```python
from build123d import *

# Parameters (mm, degrees)
F0_W     = 88.9
F0_H     = 327.66
F0_R     = 12.7
F0_R_2   = 12.7063161154
F1_DEPTH = 0.5
F2_DEPTH = 0.005
F3_R     = 5.08
F4_R     = 5.08


# Not quite as in the source:
# - a feature names something its author has since deleted; it is built from what else it names


with BuildPart() as f1:
    # F0 (on Top) → F1 (new body)
    with BuildSketch(Plane.XY):
        with Locations((-16.0019993782, 26.0465461761)):
            Rectangle(F0_W, F0_H)
        with Locations((5.5880006218, -113.6534538239)):
            Circle(F0_R, mode=Mode.SUBTRACT)
        with Locations((-37.5932163954, 166.1064843748)):
            Circle(F0_R_2, mode=Mode.SUBTRACT)
        with BuildLine():
            ThreePointArc((5.589217639, 178.8128004902), (14.573939928, 175.0912066639), (18.2955337543, 166.1064843748))
            Line((18.2955337543, 166.1064843748), (18.2955337543, -96.8894538239))
            Line((18.2955337543, -96.8894538239), (-11.1759993782, -96.8894538239))
            Line((-11.1759993782, -96.8894538239), (-11.1759993782, -126.3534538239))
            Line((-11.1759993782, -126.3534538239), (-37.5919993782, -126.3534538239))
            ThreePointArc((-37.5919993782, -126.3534538239), (-46.5722554993, -122.633709945), (-50.2919993782, -113.6534538239))
            Line((-50.2919993782, -113.6534538239), (-50.2919993782, 149.3424895761))
            Line((-50.2919993782, 149.3424895761), (-20.826782361, 149.3424895761))
            Line((-20.826782361, 149.3424895761), (-20.826782361, 178.8128004902))
            Line((-20.826782361, 178.8128004902), (5.589217639, 178.8128004902))
        make_face(mode=Mode.SUBTRACT)
    extrude(amount=F1_DEPTH)

    # F0 (on Top) → F2 (join)
    with BuildSketch(Plane.XY):
        with BuildLine():
            Line((18.2955337543, -96.8894538239), (18.2955337543, 166.1064843748))
            ThreePointArc((18.2955337543, 166.1064843748), (-3.3955046501, 157.1217620858), (5.589217639, 178.8128004902))
            Line((5.589217639, 178.8128004902), (-20.826782361, 178.8128004902))
            Line((-20.826782361, 178.8128004902), (-20.826782361, 149.3424895761))
            Line((-20.826782361, 149.3424895761), (-50.2919993782, 149.3424895761))
            Line((-50.2919993782, 149.3424895761), (-50.2919993782, -113.6534538239))
            ThreePointArc((-50.2919993782, -113.6534538239), (-37.5919993782, -100.9534538239), (-24.8919993782, -113.6534538239))
            ThreePointArc((-24.8919993782, -113.6534538239), (-28.6117432571, -122.633709945), (-37.5919993782, -126.3534538239))
            Line((-37.5919993782, -126.3534538239), (-11.1759993782, -126.3534538239))
            Line((-11.1759993782, -126.3534538239), (-11.1759993782, -96.8894538239))
            Line((-11.1759993782, -96.8894538239), (18.2955337543, -96.8894538239))
        make_face()
    extrude(amount=F2_DEPTH)

    # F3
    f3_edges = [f1.edges().sort_by_distance(p)[0] for p in [
        (28.448001, 189.876546, 0.25),
        (-60.451999, 189.876546, 0.25),
        (-60.451999, -137.783454, 0.25),
        (28.448001, -137.783454, 0.25),
        (18.295534, -96.889454, 0.2525),
        (-11.175999, -96.889454, 0.2525),
        (-11.175999, -126.353454, 0.2525),
    ]]
    fillet(f3_edges, radius=F3_R)

    # F4
    f4_edges = [f1.edges().sort_by_distance(p)[0] for p in [
        (-20.826782, 149.34249, 0.2525),
        (-50.291999, 149.34249, 0.2525),
        (-20.826782, 178.8128, 0.2525),
    ]]
    fillet(f4_edges, radius=F4_R)


solid = f1.part
```
Verification items for the finished model (mm, model axes). Give positions to 0.01 mm unless a question says otherwise; leave off trailing zeros. Order: outer loops, then holes, each group sorted by start corner. A loop starts at its lowest first (then second) coordinate and runs counter-clockwise, first axis right, second up. Notation, with made-up numbers: (82.5, 81) - (109.5, 81) arc R34 cw to (109.5, 115) - close; hole circle Ø3 at (-19.5, -32). An arc over 180 degrees is marked (long way). Answer as CSV lines item,"result". Start each with the question number.
Item 1: Section check C-C, the plane y = -105.5. Record the boundary of the cut face in (x, z) (3 decimals).
Item 2: Section check A-A, the plane z = 0.35. Record the boundary of the cut face in (x, y), plus the area to 3 significant figures.
Item 3: Mould release check, pull along X, two halves, no side actions. Record for faces 1 (the face through (3.935, -101.062, 0.246)), 2 (the face through (20, 39, 0.5)): released by +X, released by -X, zero draft, split by the parting line, or undercut.
Item 4: Material ranges on L1, parallel to X at y = 74.5, z = 0.3; L2, parallel to Y at x = 15, z = 0.45; L3, parallel to Y at x = -29, z = 0.15, recorded low to high.
Item 5: Section check D-D, the plane y = 63. Record the boundary of the cut face in (x, z) (3 decimals).
Item 6: Section check B-B, the plane x = -3. Record the boundary of the cut face in (y, z) (3 decimals).
Item 7: Gauge pin test, flat end, axial feed: pin 1 (20.5 mm diameter, centred on x = -3, y = -39.5, fed in from +Z) (3 decimals). Record the tip position at first contact, or that the pin passes through.
Filled in:
1,outline,"(-60.452, 0) - (-47.329, 0) - (-47.329, 0.005) - (-50.292, 0.005) - (-50.292, 0.5) - (-60.452, 0.5) - close; (-27.855, 0) - (-4.149, 0) - (-4.149, 0.5) - (-11.176, 0.5) - (-11.176, 0.005) - (-27.855, 0.005) - close; (15.325, 0) - (28.448, 0) - (28.448, 0.5) - (15.325, 0.5) - close"
2,outline,"(-60.45, -132.7) arc R5.08 ccw to (-55.37, -137.78) - (23.37, -137.78) arc R5.08 ccw to (28.45, -132.7) - (28.45, 184.8) arc R5.08 ccw to (23.37, 189.88) - (-55.37, 189.88) arc R5.08 ccw to (-60.45, 184.8) - close; hole circle Ø25.41 at (-37.59, 166.11); hole (-50.29, -113.65) arc R12.7 ccw to (-37.59, -126.35) - (-16.26, -126.35) arc R5.08 ccw to (-11.18, -121.27) - (-11.18, -101.97) arc R5.08 cw to (-6.1, -96.89) - (13.22, -96.89) arc R5.08 ccw to (18.3, -91.81) - (18.3, 166.11) arc R12.71 ccw to (5.59, 178.81) - (-15.75, 178.81) arc R5.08 ccw to (-20.83, 173.73) - (-20.83, 154.42) arc R5.08 cw to (-25.91, 149.34) - (-45.21, 149.34) arc R5.08 ccw to (-50.29, 144.26) - close; hole circle Ø25.4 at (5.59, -113.65)"
2,area,"8,980 mm^2"
3,face 1,"undercut"
3,face 2,"zero draft"
4,L1,"-60.45 to -50.29, 18.3 to 28.45"
4,L2,"-137.78 to -122.18, -105.13 to -96.57, 174.64 to 189.88"
4,L3,"-137.78 to -126.35, 149.34 to 156.75, 175.47 to 189.88"
5,outline,"(-60.452, 0) - (28.448, 0) - (28.448, 0.5) - (18.296, 0.5) - (18.296, 0.005) - (-50.292, 0.005) - (-50.292, 0.5) - (-60.452, 0.5) - close"
6,outline,"(-137.783, 0) - (-123.01, 0) - (-123.01, 0.5) - (-137.783, 0.5) - close; (-104.297, 0) - (156.743, 0) - (156.743, 0.005) - (-96.889, 0.005) - (-96.889, 0.5) - (-104.297, 0.5) - close; (175.47, 0) - (189.877, 0) - (189.877, 0.5) - (178.813, 0.5) - (178.813, 0.005) - (175.47, 0.005) - close"
7,pin 1,"z = 0.005"
